```python
from build123d import *

# Parameters (mm, degrees)
SKETCH2_R           = 4.755
BOSS_EXTRUDE1_DEPTH = 3
SKETCH3_R           = 4.755
BOSS_EXTRUDE2_DEPTH = 45


with BuildPart() as part:
    # Sketch1 → Revolve1 (revolve)
    with BuildSketch(Plane.XY):
        with BuildLine():
            Line((0, 0), (0, 15))
            ThreePointArc((0, 15), (-7.5, 7.5), (0, 0))
        make_face()
    revolve(axis=Axis((0, 0, 0), (0, 1, 0)))

    # Sketch2 → Boss-Extrude1 (add)
    with BuildSketch(Plane(origin=(0, 0, 0), x_dir=(-1, 0, 0), z_dir=(0, -1, 0))):
        Circle(SKETCH2_R)
    extrude(amount=-BOSS_EXTRUDE1_DEPTH)

    # Sketch3 → Boss-Extrude2 (add)
    with BuildSketch(Plane(origin=(0, 0, 0), x_dir=(-1, 0, 0), z_dir=(0, -1, 0))):
        Circle(SKETCH3_R)
    extrude(amount=BOSS_EXTRUDE2_DEPTH)


solid = part.part
```
Geometry check sheet. Reference: the model listing, model coordinates, mm. A direction names the side the tool comes from. Round coordinates to 2 decimals unless told otherwise and drop trailing zeros. Write each loop counter-clockwise with the first axis right and the second up, starting at its lowest first coordinate (ties: lowest second). Pieces come first, ordered by that corner, then holes. Notation, with made-up numbers: (-29, 53.25) -> (11, 53.25) arc R22 ccw to (11, 59.25) -> close; hole circle Ø8 at (75.25, 44). An arc over 180 degrees is marked (long way). Put each result on its own line as item: value.
1) Cross-section at B-B, the plane x = 0. Enter the section's corners in (y, z) (3 decimals).
Recorded:
outline: (-45, -4.755) -> (1.7, -4.755) arc R7.5 ccw (long way) to (1.7, 4.755) -> (-45, 4.755) -> close
2) Thickness scan on probe 1 along Z at (x, y) = (0, -41.5) (3 decimals); probe 2 along Z at (x, y) = (-4.5, 2). Record the ranges inside material, lowest first. Write a range as from..to.
Recorded:
probe 1: z = -4.755..4.755
probe 2: z = -2.4..2.4
3) Cross-section at A-A, the plane y = -9. Enter the section's corners in (x, z) (3 decimals).
Recorded:
outline: circle Ø9.51 at (0, 0)
4) Cross-section at C-C, the plane z = 0. Enter the section's corners in (x, y) (3 decimals), plus the area to 3 significant figures.
Recorded:
outline: (-4.755, -45) -> (4.755, -45) -> (4.755, 1.7) arc R7.5 ccw (long way) to (-4.755, 1.7) -> close
area: 610 mm2
5) Depth check by flat-ended pin: P1, Ø5, axis at x = -1.5, y = -17.5, coming from the -Z side (3 decimals); P2, Ø2, axis at x = -5, z = -2, coming from the -Y side; P3, Ø1, axis at x = 4, y = 0, coming from the -Z side; P4, Ø3, axis at x = 5.5, y = -18, coming from the +Z side. Enter the tip coordinate at first touch or a pass-through.
Recorded:
P1: stops at z = -4.755
P2: stops at y = -45
P3: stops at z = -3.22
P4: stops at z = 2.57
6) Access from +Z, -Z, +X, -X, +Y, -Y to the whole of each face (thin tool, end or side, straight path). Record for faces 1 (the face through (-4.535, -21.323, -1.428)), 2 (the face through (0, -45, 0)).
Recorded:
face 1: -Y
face 2: +Z, -Z, +X, -X, -Y
